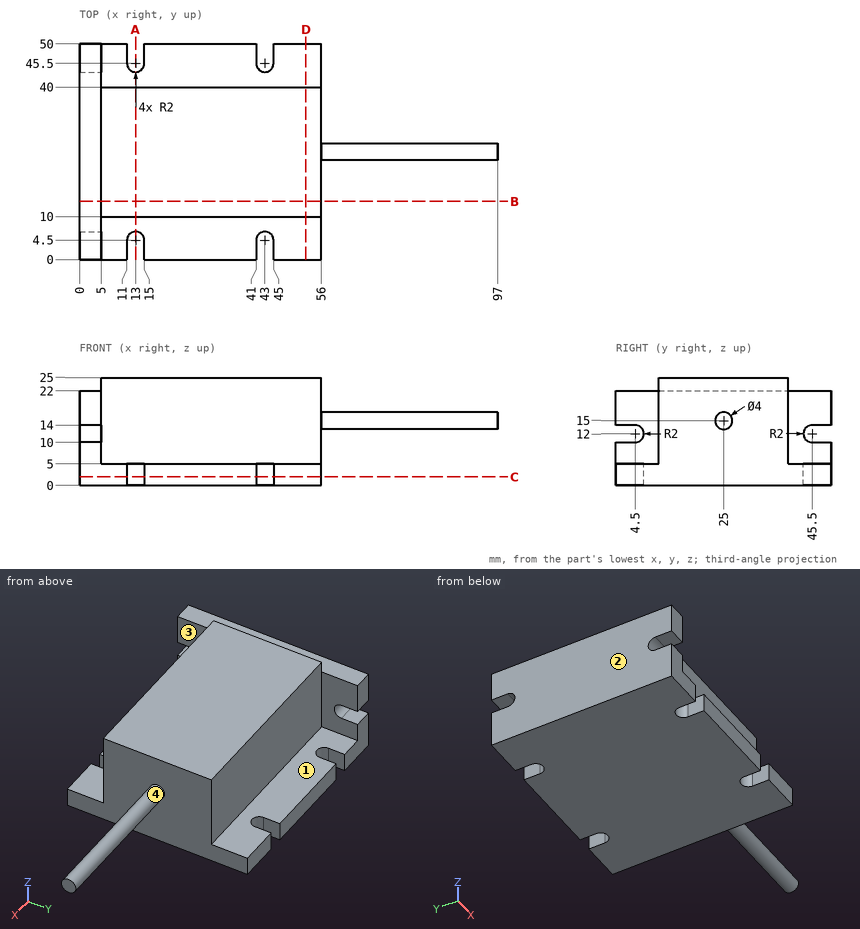
Input: dimensioned drawing with shaded views. Units: mm. Origin: part minimum x, y, z. A direction names the side the tool comes from. Give positions to 0.01 mm unless a question says otherwise; leave off trailing zeros. Loops run counter-clockwise (first coordinate to the right, second up) from the corner with the lowest first, then second, coordinate; pieces in that order, holes last. Notation, with made-up numbers: (-21.5, -27.75) -> (-1.5, -27.75) arc R24 cw to (-1.5, 5.25) -> close; hole circle Ø6 at (85, -23). An arc over 180 degrees is marked (long way). Use a Markdown table: item, result. Add a question column.
1) Line query: line 1 along Y through (x, z) = (6.5, 8); line 2 along X through (y, z) = (23.5, 19.25); line 3 along Y through (x, z) = (69, 15.25). Output: solid intervals per line, ascending. Write a range as [from, to].
2) Section query A-A, the plane x = 13. Return the cut outline in (y, z).
3) Reachability of the marked faces 1, 2, 3 and 4 from +Z, -Z, +X, -X, +Y, -Y: full face, straight path, thin tool, end or side. Return the list, or none.
4) First-contact query: pin 1 (2 mm diameter, centred on y = 48.5, z = 3.5, fed in from +X); pin 2 (2 mm diameter, centred on x = 52, z = 21, fed in from -Y); pin 3 (4 mm diameter, centred on x = 26, y = 43, fed in from +Z). Flat tips, straight axial feed; report the tip coordinate or a pass-through.
5) Section query C-C, the plane z = 2. Return the cut outline in (x, y).
6) Section query B-B, the plane y = 13.5. Return the cut outline in (x, z).
7) Section query D-D, the plane x = 52.5. Return the cut outline in (y, z).
Numbers:
| question | item | result |
|---|---|---|
| 1 | line 1 | y = [10, 40] |
| 1 | line 2 | x = [0, 56] |
| 1 | line 3 | y = [23.02, 26.98] |
| 2 | outline | (6.5, 0) -> (43.5, 0) -> (43.5, 5) -> (40, 5) -> (40, 25) -> (10, 25) -> (10, 5) -> (6.5, 5) -> close |
| 3 | face 1 | +Z, +X, +Y |
| 3 | face 2 | +Z, -Z, -X, +Y, -Y |
| 3 | face 3 | +Z, +X, -Y |
| 3 | face 4 | +X |
| 4 | pin 1 | stops at x = 56 |
| 4 | pin 2 | stops at y = 10 |
| 4 | pin 3 | stops at z = 5 |
| 5 | outline | (0, 0) -> (11, 0) -> (11, 4.5) arc R2 cw to (15, 4.5) -> (15, 0) -> (41, 0) -> (41, 4.5) arc R2 cw to (45, 4.5) -> (45, 0) -> (56, 0) -> (56, 50) -> (45, 50) -> (45, 45.5) arc R2 cw to (41, 45.5) -> (41, 50) -> (15, 50) -> (15, 45.5) arc R2 cw to (11, 45.5) -> (11, 50) -> (0, 50) -> close |
| 6 | outline | (0, 0) -> (56, 0) -> (56, 25) -> (5, 25) -> (5, 22) -> (0, 22) -> close |
| 7 | outline | (0, 0) -> (50, 0) -> (50, 5) -> (40, 5) -> (40, 25) -> (10, 25) -> (10, 5) -> (0, 5) -> close |
